Job drawing, mm, ordinate dimensions from the low corner. One solid piece. A direction names the side the tool comes from. Coordinates: 2 decimals unless noted, no trailing zeros. Write each loop counter-clockwise with the first axis right and the second up, starting at its lowest first coordinate (ties: lowest second). Pieces come first, ordered by that corner, then holes. Notation, with made-up numbers: (-23, 76.25) - (-2, 76.25) arc R28 cw to (-2, 104.25) - close; hole circle Ø10 at (-12.75, 88). An arc over 180 degrees is marked (long way). Use a Markdown table: item, result.
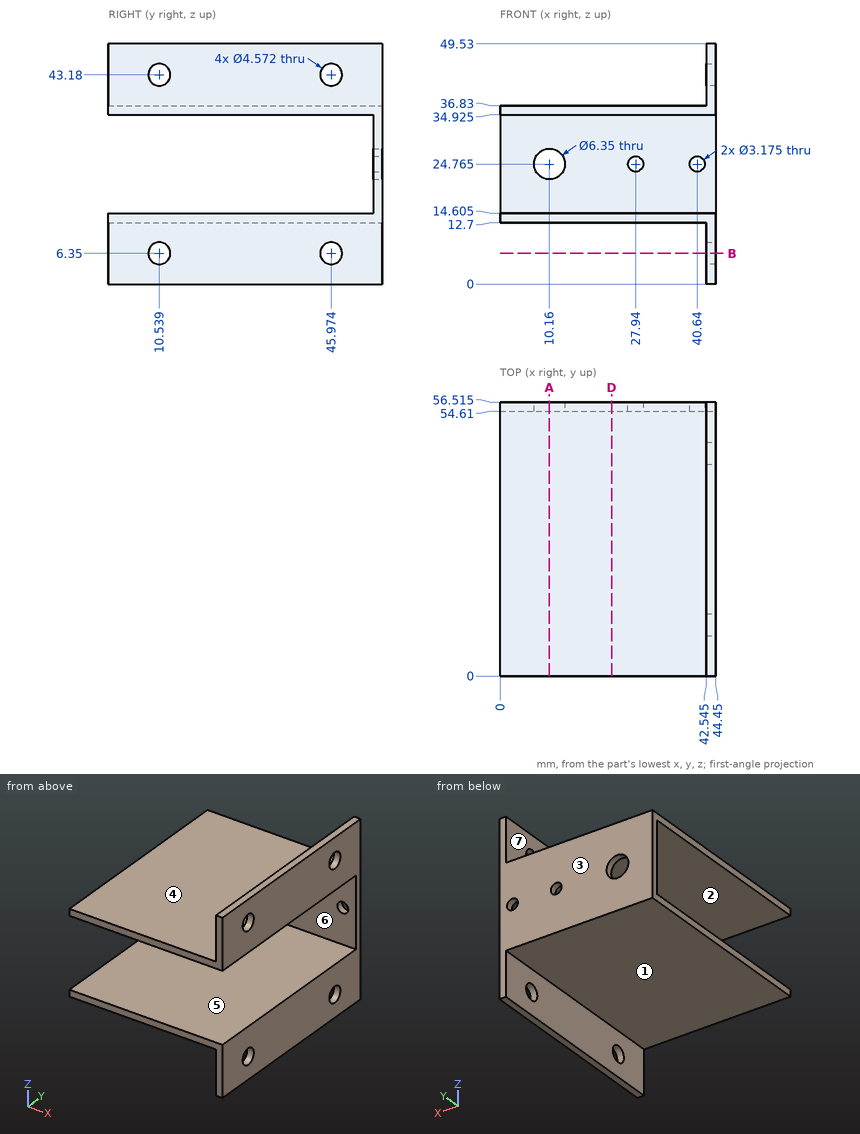
Item 1: Drill centre lines: probe 1 along Y at (x, z) = (44.05, 43.18) (1 decimal); probe 2 along Z at (x, y) = (27.94, 56.05); probe 3 along Z at (x, y) = (42.5, 17) (1 decimal). Where is each one in solid material? Low to high.
From the geometry:
| item | result |
|---|---|
| probe 1 | 0 to 8.3, 12.8 to 43.7, 48.3 to 56.5 |
| probe 2 | 12.7 to 23.18, 26.35 to 36.83 |
| probe 3 | 12.7 to 14.6, 34.9 to 36.8 |
Item 2: Band-saw the part on A-A, the plane x = 10.16. Give the cut face in (y, z) (1 decimal), then the cut area to 3 significant figures.
From the geometry:
| item | result |
|---|---|
| outline | (0, 12.7) - (56.5, 12.7) - (56.5, 21.6) - (54.6, 21.6) - (54.6, 14.6) - (0, 14.6) - close; (0, 34.9) - (54.6, 34.9) - (54.6, 27.9) - (56.5, 27.9) - (56.5, 36.8) - (0, 36.8) - close |
| area | 242 mm^2 |
Item 3: Drop flat-ended pins along their axis: P1, Ø6, axis at y = 8.5, z = 6, coming from the -X side (3 decimals); P2, Ø4, axis at y = 10.54, z = 43.18, coming from the -X side; P3, Ø22, axis at x = 21, y = 15, coming from the -Z side; P4, Ø13, axis at x = 24, y = 30.5, coming from the +Z side. Give the stop position or say it passes through.
From the geometry:
| item | result |
|---|---|
| P1 | x = 42.545 |
| P2 | through |
| P3 | z = 12.7 |
| P4 | z = 36.83 |
Item 4: Band-saw the part on B-B, the plane z = 6.35. Count the separate pieces of the cut face and the enclosed holes in it.
From the geometry:
| item | result |
|---|---|
| separate pieces | 3 |
| enclosed holes | 0 |
Item 5: Band-saw the part on D-D, the plane x = 23. Give the cut face in (y, z) (1 decimal), then the cut area to 3 significant figures.
From the geometry:
| item | result |
|---|---|
| outline | (0, 12.7) - (56.5, 12.7) - (56.5, 36.8) - (0, 36.8) - (0, 34.9) - (54.6, 34.9) - (54.6, 14.6) - (0, 14.6) - close |
| area | 254 mm^2 |
Item 6: Two-plate mould, pull along Z, no slides. Class the marked faces 4, 5, 6 and 7: pulls with the +Z half, pulls with the -Z half, needs draft (parallel to the pull), parting line crosses it, or undercut.
From the geometry:
| item | result |
|---|---|
| face 4 | pulls with the +Z half |
| face 5 | undercut |
| face 6 | undercut |
| face 7 | needs draft |
Item 7: Which spindle directions (+Z, -Z, +X, -X, +Y, -Y) get a long thin tool onto all of the face, cutting with end or side? Do the marked faces 1, 2 and 3. Say none if no direction does.
From the geometry:
| item | result |
|---|---|
| face 1 | -Z, -X, +Y, -Y |
| face 2 | +X, -X, -Y |
| face 3 | +Z, -Z, +X, -X, +Y |
